from build123d import *

# Parameters (mm, degrees)
BOSS_EXTRUDE1_DEPTH                         = 50.8
CBORE_FOR_5_BINDING_HEAD_MACHINE_SC_2_COUNT = 2
CBORE_FOR_5_BINDING_HEAD_MACHINE_SC_2_PITCH = 40.189879992
CBORE_FOR_5_BINDING_HEAD_MACHINE_SC_3_COUNT = 2
CBORE_FOR_5_BINDING_HEAD_MACHINE_SC_3_PITCH = 40.181482417


with BuildPart() as part:
    # Sketch1 → Boss-Extrude1 (new body)
    with BuildSketch(Plane.XY):
        with BuildLine():
            Line((41.275, -15.999909517), (41.275, -22.9235))
            Line((41.275, -22.9235), (-41.275, -22.9235))
            Line((-41.275, -22.9235), (-41.275, -16.00020267))
            Line((-41.275, -16.00020267), (-32.120446577, -16.00020267))
            ThreePointArc((-32.120446577, -16.00020267), (-26.090409627, -13.03885638), (-24.747256549, -6.456542406))
            ThreePointArc((-24.747256549, -6.456542406), (0, 25.575645574), (24.747256549, -6.456542406))
            ThreePointArc((24.747256549, -6.456542406), (26.09048422, -13.03895293), (32.120690592, -16.000202666))
            Line((32.120690592, -16.000202666), (41.275, -15.999909517))
        make_face()
        with BuildLine():
            Line((0, 14.605), (12.262196034, 14.605))
            ThreePointArc((12.262196034, 14.605), (19.070067555, 0), (12.262196034, -14.605))
            Line((12.262196034, -14.605), (0, -14.605))
            Line((0, -14.605), (-12.262196034, -14.605))
            ThreePointArc((-12.262196034, -14.605), (-19.070067555, 0), (-12.262196034, 14.605))
            Line((-12.262196034, 14.605), (0, 14.605))
        make_face(mode=Mode.SUBTRACT)
    extrude(amount=BOSS_EXTRUDE1_DEPTH)

    # Sketch6 → CBORE for #5 Binding Head Machine Screw1 (revolve, cut)
    with BuildSketch(Plane(origin=(-36.697723288, -16.00020267, 5.28577815), x_dir=(0, 0, 1), z_dir=(1, 0, 0))):
        Polygon((0, 0), (0, 6.92329733), (1.7272, 6.92329733), (1.7272, 1.9812), (3.77063, 1.9812), (3.77063, 0.635), (4.40563, 0), align=None)
    cbore_for_5_binding_head_machine_screw1 = revolve(axis=Axis((-36.697723288, -9.65020267, 5.28577815), (0, -1, 0)), mode=Mode.SUBTRACT)

    # CBORE for _5 Binding Head Machine Sc 2: CBORE for #5 Binding Head Machine Screw1 ×2
    with Locations(*[(0, 0, i * CBORE_FOR_5_BINDING_HEAD_MACHINE_SC_2_PITCH) for i in range(1, CBORE_FOR_5_BINDING_HEAD_MACHINE_SC_2_COUNT)]):
        add(cbore_for_5_binding_head_machine_screw1, mode=Mode.SUBTRACT)

    # Sketch8 → CBORE for #5 Binding Head Machine Screw2 (revolve, cut)
    with BuildSketch(Plane(origin=(36.697845296, -16.000056092, 5.268033609), x_dir=(-0.9999999994872624, -3.2023045840411235e-05, 0), z_dir=(0, 0, 1))):
        Polygon((0, 0), (0, 6.923590479), (1.7272, 6.923590479), (1.7272, 1.9812), (3.77063, 1.9812), (3.77063, 0.635), (4.40563, 0), align=None)
    cbore_for_5_binding_head_machine_screw2 = revolve(axis=Axis((36.69764195, -9.650056095, 5.268033609), (3.20230458404138e-05, -0.9999999994872623, 0)), mode=Mode.SUBTRACT)

    # CBORE for _5 Binding Head Machine Sc 3: CBORE for #5 Binding Head Machine Screw2 ×2
    with Locations(*[(0, 0, i * CBORE_FOR_5_BINDING_HEAD_MACHINE_SC_3_PITCH) for i in range(1, CBORE_FOR_5_BINDING_HEAD_MACHINE_SC_3_COUNT)]):
        add(cbore_for_5_binding_head_machine_screw2, mode=Mode.SUBTRACT)


solid = part.part
Could you check a few things on this model? Use its own coordinates, in mm. A direction names the side the tool comes from. Round coordinates to 2 decimals unless told otherwise and drop trailing zeros. Write each loop counter-clockwise with the first axis right and the second up, starting at its lowest first coordinate (ties: lowest second). Pieces come first, ordered by that corner, then holes. Notation, with made-up numbers: (75, 86) -> (106, 86) arc R35 ccw to (106, 125) -> close; hole circle Ø10 at (-8.75, 35.25). An arc over 180 degrees is marked (long way). Use a Markdown table: item, result.
1. Which directions (+Z, -Z, +X, -X, +Y, -Y) give clear straight access to the entire face, cutting with the end or side of a thin tool? Please do faces 1 (the face through (-19.07, -0.23, 25.04)), 2 (the face through (41.275, -19, 25)).
Answer key:
| item | result |
|---|---|
| face 1 | +Z, -Z |
| face 2 | +Z, -Z, +X, +Y, -Y |
2. We'd pull the mould along Z, two halves only. Please class faces 3 (the face through (-38, -17.981, 44)), 4 (the face through (-35.647, -20.418, 44.105)), 5 (the face through (-0.654, 25.567, 25.044)), 6 (the face through (3, -15, 0)): +Z half, -Z half, draft (parallel to the pull), parting line (faces both ways), or undercut.
Answer key:
| item | result |
|---|---|
| face 3 | undercut |
| face 4 | undercut |
| face 5 | draft |
| face 6 | -Z half |
3. If we section it at C-C (z = 31): List the corners of the cut face in (x, y) for me (1 decimal).
Answer key:
| item | result |
|---|---|
| outline | (-41.3, -22.9) -> (41.3, -22.9) -> (41.3, -16) -> (32.1, -16) arc R7.6 cw to (24.7, -6.5) arc R25.6 ccw (long way) to (-24.7, -6.5) arc R7.6 cw to (-32.1, -16) -> (-41.3, -16) -> close; hole (-12.3, -14.6) -> (12.3, -14.6) arc R19.1 ccw to (12.3, 14.6) -> (-12.3, 14.6) arc R19.1 ccw to start |
4. If we section it at D-D (x = 28.5): List the corners of the cut face in (y, z) for me, then the cut area to 3 significant figures.
Answer key:
| item | result |
|---|---|
| outline | (-22.92, 0) -> (-15.09, 0) -> (-15.09, 50.8) -> (-22.92, 50.8) -> close |
| area | 398 mm^2 |
5. If we section it at B-B (y = -4.5): List the corners of the cut face in (x, z) for me.
Answer key:
| item | result |
|---|---|
| outline | (-25.18, 0) -> (-18.53, 0) -> (-18.53, 50.8) -> (-25.18, 50.8) -> close; (18.53, 0) -> (25.18, 0) -> (25.18, 50.8) -> (18.53, 50.8) -> close |
6. Please list where these lines run through material, in increasing order: probe 1 along X at (y, z) = (-17, 43) (1 decimal); probe 2 along Y at (x, z) = (38, 19.5); probe 3 along X at (y, z) = (14.5, 11.5).
Answer key:
| item | result |
|---|---|
| probe 1 | x = -41.3 to -39.5, -33.9 to 33.8, 39.6 to 41.3 |
| probe 2 | y = -22.92 to -16 |
| probe 3 | x = -21.07 to -12.39, 12.39 to 21.07 |
7. For pin 1 Ø12.5 at (x, z) = (-5, 19) entering from +Y; pin 2 Ø10 at (x, z) = (36.5, 25.5) entering from +Y; pin 3 Ø2 at (x, z) = (-36.7, 5.29) entering from +Y; pin 4 Ø4 at (x, z) = (-37.5, 43.5) entering from +Y, each with a flat end and sliding along its axis, tell me the tip position at first contact or that it passes through.
Answer key:
| item | result |
|---|---|
| pin 1 | stops at y = 25.58 |
| pin 2 | stops at y = -15.97 |
| pin 3 | passes through |
| pin 4 | stops at y = -16.27 |
8. If we section it at A-A (x = 0): List the corners of the cut face in (y, z) for me (1 decimal), then the cut area to 3 significant figures.
Answer key:
| item | result |
|---|---|
| outline | (-22.9, 0) -> (-14.6, 0) -> (-14.6, 50.8) -> (-22.9, 50.8) -> close; (14.6, 0) -> (25.6, 0) -> (25.6, 50.8) -> (14.6, 50.8) -> close |
| area | 980 mm^2 |
